Can you work these out from the model? Positions are in its coordinate system, mm. A direction names the side the tool comes from. Coordinates: 2 decimals unless noted, no trailing zeros. Order: outer loops, then holes, each group sorted by start corner. A loop starts at its lowest first (then second) coordinate and runs counter-clockwise, first axis right, second up. Notation, with made-up numbers: (57, 19) -> (68, 19) arc R17 ccw to (68, 48) -> close; hole circle Ø3 at (-33, 67.25). An arc over 180 degrees is marked (long way). Answer in a Markdown table with one row per item. Add a question column.
1. On a 3-axis mill with a long thin cutter (end or side, diameter ignored), from which of +Z, -Z, +X, -X, +Y, -Y can I reach the whole of each face in a straight line? I mean faces 4 (the face through (0.031, -10.764, -1.507)), 5 (the face through (-2, 0, 0)), 6 (the face through (0.031, -10.764, 1.493)). Say none if no direction works.
2. If I drill on line 1 along Y through (x, z) = (0, -0.45); line 2 along Y through (x, z) = (0.95, 0.4); line 3 along X through (y, z) = (-15, 0.1), over which ranges is the centre line in solid material (lowest first)? Write a range as [from, to].
3. We'd pull the mould along Y, two halves only. Please class faces 1 (the face through (-0.16, 13.76, -0.03)), 2 (the face through (0, -17, 0)), 3 (the face through (0, 3, 2)): pulls with the +Y half, pulls with the -Y half, needs draft (parallel to the pull), parting line crosses it, or undercut.
4. Imagine slicing it at B-B on z = -0.15. Write out the boundary of the cut face in (x, y).
5. Will these pins go through, and if not, where does the flat tip stop? pin 1 (2 mm diameter, centred on x = -1, y = -12.5, fed in from -Z); pin 2 (1.2 mm diameter, centred on x = 1, y = -13.5, fed in from +Z).
6. Imagine slicing it at A-A on x = 0. Write out the boundary of the cut face in (y, z), plus the area to 3 significant figures.
Autodesk Inventor part; units mm, degrees
ref_plane "YZ Plane" through (0, 0, 0) normal (1, 0, 0) x (0, 1, 0)
ref_plane "XZ Plane" through (0, 0, 0) normal (0, 1, 0) x (-1, 0, 0)
ref_plane "XY Plane" through (0, 0, 0) normal (0, 0, 1) x (1, 0, 0)
sketch "Sketch6" plane through (0, 0, 0) normal (0, 0, 1) x (1, 0, 0)
  line L0 (0, 0) -> (0, 15)
  line L1 (0, 15) -> (2, 15)
  line L2 (2, 15) -> (-2, 15)
  line L3 (-2, 15) -> (-2, -15)
  line L4 (-2, -15) -> (2, -15)
  line L5 (2, -15) -> (2, 15)
  circle A0 centre (0, 15) radius 1.25
  circle A1 centre (0, 15) radius 2
  circle A2 centre (0, -15) radius 1.25
  circle A3 centre (0, -15) radius 2
  line L6 (-2, -15) -> (-2, -10)
  line L7 (2, -15) -> (2, -10)
  line L8 (-2, 15) -> (2, 15)
  line L9 (2, 15) -> (2, 14)
  line L10 (2, 14) -> (-2, 14)
  line L11 (-2, 14) -> (-2, 15)
  arc A4 (-2, 14) -> (2, 14) centre (0, 14) ccw
  arc A5 (-2, -10) -> (2, -10) centre (0, -7.7639) ccw
  point P0 (-2, 14)
  point P1 (0, 12)
  point P2 (0, 13.75)
  point P3 (1.25, 15)
  dimension "d115" = 15
  dimension "d116" = 2
  dimension "d117" = 4
  dimension "d118" = 30
  dimension "d119" = 2.5
  dimension "d120" = 2.5
  dimension "d122" = 5
  dimension "d124" = 1
  dimension "d125" = 2
  dimension "d132" = 3
  dimension "d133" = 5
extrude "Extrusion8" add sketch "Sketch6" along normal mid plane 4 contours A4 L10 A1 L0 | A4 L5 A5 L3 | L0 A1 L10 A4 | A1 L10 A0 L0 | L0 A0 L10 A1 | L3 A1 L10 | L10 A1 L5 | A1 L2 A0 L10 | L10 A0 L1 A1 | A1 L1 A0 L2
extrude "Extrusion9" cut sketch "Sketch6" along normal mid plane 2 contours A3 L4 A2 | L4 A2 A3
extrude "Extrusion10" add sketch "Sketch6" along normal mid plane 2 contours A5 L5 A3 L3 | A3 L4 A2 | L4 A2 A3
properties part number "link7" material "Aluminum 6061"
Answers follow:
| question | item | result |
|---|---|---|
| 1 | face 4 | -Z, -Y |
| 1 | face 5 | +Z, -Z, -X, +Y, -Y |
| 1 | face 6 | +Z, -Y |
| 2 | line 1 | y = [-17, -16.25], [-13.75, 13.75], [16.25, 17] |
| 2 | line 2 | y = [-16.76, -15.81], [-14.19, 14.19], [15.81, 16.76] |
| 2 | line 3 | x = [-2, -1.25], [1.25, 2] |
| 3 | face 1 | undercut |
| 3 | face 2 | pulls with the -Y half |
| 3 | face 3 | needs draft |
| 4 | outline | (-2, -15) arc R2 ccw to (2, -15) -> (2, 15) arc R2 ccw to (-2, 15) -> close; hole circle Ø2.5 at (0, -15); hole circle Ø2.5 at (0, 15) |
| 5 | pin 1 | stops at z = -1 |
| 5 | pin 2 | stops at z = 1 |
| 6 | outline | (-17, -1) -> (-16.25, -1) -> (-16.25, 1) -> (-17, 1) -> close; (-13.75, -1) -> (-10.76, -1) -> (-10.76, -2) -> (13.75, -2) -> (13.75, 2) -> (-10.76, 2) -> (-10.76, 1) -> (-13.75, 1) -> close; (16.25, -2) -> (17, -2) -> (17, 2) -> (16.25, 2) -> close |
| 6 | area | 109 mm² |
